from build123d import *

# Parameters (mm, degrees)
F0_R     = 3
F1_DEPTH = 0.4
F2_R     = 1.95
F3_DEPTH = 2.5
F4_R     = 1.45
F5_DEPTH = 2.1
F6_R     = 0.75
F7_DEPTH = 2


with BuildPart() as f1:
    # F0 (on Top) → F1 (new body)
    with BuildSketch(Plane.XY):
        Circle(F0_R)
    extrude(amount=F1_DEPTH)

    # F2 (on face) → F3 (join)
    with BuildSketch(Plane(origin=(0, 0, 0), x_dir=(1, 0, 0), z_dir=(0, 0, -1))):
        Circle(F2_R)
    extrude(amount=F3_DEPTH)

    # F4 (on face) → F5 (join)
    with BuildSketch(Plane(origin=(0, 0, -2.5), x_dir=(1, 0, 0), z_dir=(0, 0, -1))):
        Circle(F4_R)
    extrude(amount=F5_DEPTH)

    # F6 (on face) → F7 (cut)
    with BuildSketch(Plane(origin=(0, 0, -4.6), x_dir=(1, 0, 0), z_dir=(0, 0, -1))):
        Circle(F6_R)
    extrude(amount=-F7_DEPTH, mode=Mode.SUBTRACT)


solid = f1.part
Model file for the job. Use its own axes, mm. A direction names the side the tool comes from. Give positions to 0.01 mm unless a question says otherwise; leave off trailing zeros. Loops run counter-clockwise (first coordinate to the right, second up) from the corner with the lowest first, then second, coordinate; pieces in that order, holes last. Notation, with made-up numbers: (-11, 38.25) -> (-4, 38.25) arc R18 ccw to (-4, 44.25) -> close; hole circle Ø10 at (72.25, 82). An arc over 180 degrees is marked (long way). Use a Markdown table: item, result. Add a question column.
(1) Slice it at C-C on z = -2.8. List the corners of the cut face in (x, y), and give its area (3 significant figures).
(2) Drop a flat-ended pin along its axis: pin 1 Ø2 at (x, z) = (1.5, -2.5) entering from -Y. Give the stop position or say it passes through.
(3) Slice it at D-D on z = -0.4. List the corners of the cut face in (x, y).
(4) Slice it at A-A on x = 0. List the corners of the cut face in (y, z), and give its area (3 significant figures).
(5) Tool access for faces 5 (the cylindrical face through (-3, 0.1, 0.2)), 6 (the cylindrical face through (-1.45, -0.06, -3.54)): list every direction of +Z, -Z, +X, -X, +Y, -Y with a clear straight run to the whole face (end or side of a thin tool).
(6) Wall check: line 1 along Y through (x, z) = (0, -3.25); line 2 along Z through (x, y) = (-2.4, 0.7). Give the ranges that are in metal, low to high.
(7) Mould opens along Y. For faces 1 (the cylindrical face through (-0.75, -0.03, -3.61)), 2 (the flat face through (0, 0, -2.6)), 3 (the flat face through (0, 0, 0.4)), 4 (the cylindrical face through (-1.437, -1.318, -1.232)) say: +Y half, -Y half, draft (parallel to the pull), parting line (faces both ways), or undercut.
Filled sheet:
| question | item | result |
|---|---|---|
| 1 | outline | circle Ø2.9 at (0, 0); hole circle Ø1.5 at (0, 0) |
| 1 | area | 4.84 mm2 |
| 2 | pin 1 | y = -1.88 |
| 3 | outline | circle Ø3.9 at (0, 0) |
| 4 | outline | (-3, 0) -> (-1.95, 0) -> (-1.95, -2.5) -> (-1.45, -2.5) -> (-1.45, -4.6) -> (-0.75, -4.6) -> (-0.75, -2.6) -> (0.75, -2.6) -> (0.75, -4.6) -> (1.45, -4.6) -> (1.45, -2.5) -> (1.95, -2.5) -> (1.95, 0) -> (3, 0) -> (3, 0.4) -> (-3, 0.4) -> close |
| 4 | area | 15.2 mm2 |
| 5 | face 5 | +Z, -Z |
| 5 | face 6 | -Z |
| 6 | line 1 | -1.45 to -0.75, 0.75 to 1.45 |
| 6 | line 2 | 0 to 0.4 |
| 7 | face 1 | undercut |
| 7 | face 2 | undercut |
| 7 | face 3 | draft |
| 7 | face 4 | parting line |
